Verification items for the finished model (mm, model axes). Give positions to 0.01 mm unless a question says otherwise; leave off trailing zeros. Order: outer loops, then holes, each group sorted by start corner. A loop starts at its lowest first (then second) coordinate and runs counter-clockwise, first axis right, second up. Notation, with made-up numbers: (73, 2.25) -> (83, 2.25) arc R12 ccw to (83, 24.25) -> close; hole circle Ø6 at (-34, 70). An arc over 180 degrees is marked (long way). Return JSON: item names as keys, results as strings. Group by question number.
(1) Thickness scan on line 1 along X through (y, z) = (-22, 4.45); line 2 along Y through (x, z) = (-63.5, 3.35); line 3 along Y through (x, z) = (-162, 1.05). Record the ranges inside material, lowest first.
(2) Cross-section at A-A on y = -26.5. Enter the section's corners in (x, z), then the cut area to 3 significant figures.
(3) Cross-section at C-C on y = 51.5. Enter the section's corners in (x, z).
(4) Depth check by flat-ended pin: pin 1 Ø3 at (x, z) = (-113.5, 4) entering from -Y; pin 2 Ø2 at (y, z) = (144.5, 1) entering from -X; pin 3 Ø3 at (y, z) = (-22.5, 2) entering from -X. Enter the tip coordinate at first touch or a pass-through.
(5) Cross-section at D-D on y = 178. Enter the section's corners in (x, z), then the cut area to 3 significant figures.
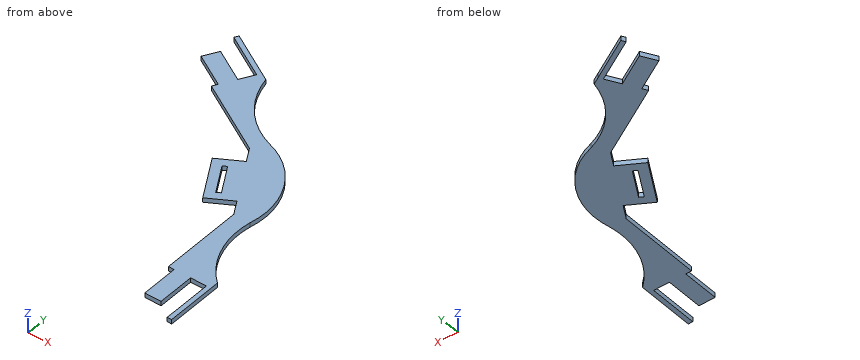
Autodesk Inventor part; units mm, degrees
ref_plane "YZ Plane" through (0, 0, 0) normal (1, 0, 0) x (0, 1, 0)
ref_plane "XZ Plane" through (0, 0, 0) normal (0, 1, 0) x (-1, 0, 0)
ref_plane "XY Plane" through (0, 0, 0) normal (0, 0, 1) x (1, 0, 0)
sketch "Sketch1" plane through (0, 0, 0) normal (0, 0, 1) x (1, 0, 0)
  arc A0 (20, 100) -> (52, 10) centre (115.8042, 83.3748) ccw
  line L0 (-10, 117.3205) -> (-38.5788, 100.8205)
  line L1 (-38.5788, 100.8205) -> (-68.5788, 152.782)
  line L2 (-68.5788, 152.782) -> (-40, 169.282)
  line L3 (-29.2894, 117.7308) -> (-34.0526, 114.9808)
  line L4 (-34.0526, 114.9808) -> (-54.0526, 149.6218)
  line L5 (-54.0526, 149.6218) -> (-49.2894, 152.3718)
  line L6 (-49.2894, 152.3718) -> (-29.2894, 117.7308)
  line L7 (-136.6025, 236.6025) -> (-50, 186.6025)
  arc A1 (-101.9423, 276.6359) -> (-40, 203.923) centre (-6.4957, 295.2045) ccw
  line L8 (-136.6025, 236.6025) -> (-50, 186.6025)
  arc A2 (20, 100) -> (-40, 203.923) centre (-65.07, 120.1668) ccw
  line L9 (-10, 117.3205) -> (0, 100)
  line L10 (-40, 169.282) -> (-50, 186.6025)
  line L11 (0, 100) -> (0, 0)
  line L12 (52, 10) -> (52, 0)
  line L13 (-110.6025, 281.6359) -> (-101.9423, 276.6359)
  line L14 (46.5, 0) -> (27.071, 0)
  line L15 (7.071, 0) -> (0, 0)
  line L16 (-136.6025, 236.6025) -> (-133.067, 242.7262)
  line L17 (-136.6025, 236.6025) -> (-129.5315, 236.6025) construction
  line L18 (-123.067, 260.0467) -> (-113.3525, 276.8727)
  line L19 (7.071, 0) -> (7.071, -45)
  line L20 (7.071, -45) -> (27.071, -45)
  line L21 (27.071, -45) -> (27.071, 0)
  line L22 (46.5, 0) -> (46.5, -60)
  line L23 (46.5, -60) -> (52, -60)
  line L24 (52, -60) -> (52, 0)
  line L25 (-110.6025, 281.6359) -> (-149.5737, 304.1359)
  line L26 (-152.3237, 299.3727) -> (-113.3525, 276.8727)
  line L27 (-123.067, 260.0467) -> (-162.0382, 282.5467)
  line L28 (-162.0382, 282.5467) -> (-172.0382, 265.2262)
  line L29 (-172.0382, 265.2262) -> (-133.067, 242.7262)
  line L30 (-149.5737, 304.1359) -> (-162.5641, 311.6359)
  line L31 (-162.5641, 311.6359) -> (-165.3141, 306.8727)
  line L32 (-165.3141, 306.8727) -> (-152.3237, 299.3727)
  dimension "d9" = 33
  dimension "d10" = 60
  dimension "d11" = 5.5
  dimension "d12" = 40
  dimension "d13" = 52
  dimension "d14" = 100
  dimension "d28" = 19.429
  dimension "d34" = 60
  dimension "d39" = 19.429
  dimension "d43" = 45
  dimension "d44" = 60
extrude "Extrusion2" add sketch "Sketch1" along normal blind 5.5
properties part number "brazos"
Verdict:
{
 "1": {"line 1": "7.07 to 27.07, 46.5 to 52", "line 2": "143.99 to 155.71, 194.4 to 216.43", "line 3": "259.43 to 282.52, 304.96 to 311.31"},
 "2": {"outline": "(7.07, 0) -> (27.07, 0) -> (27.07, 5.5) -> (7.07, 5.5) -> close; (46.5, 0) -> (52, 0) -> (52, 5.5) -> (46.5, 5.5) -> close", "area": "140 mm²"},
 "3": {"outline": "(0, 0) -> (23.94, 0) -> (23.94, 5.5) -> (0, 5.5) -> close"},
 "4": {"pin 1": "y = 222.4", "pin 2": "x = -64.37", "pin 3": "x = 7.07"},
 "5": {"outline": "(-45.03, 0) -> (0.5, 0) -> (0.5, 5.5) -> (-45.03, 5.5) -> close", "area": "250 mm²"}
}
